Build history of the part. All positions in model axes, mm. A direction names the side the tool comes from. Give positions to 0.01 mm unless a question says otherwise; leave off trailing zeros. Order: outer loops, then holes, each group sorted by start corner. A loop starts at its lowest first (then second) coordinate and runs counter-clockwise, first axis right, second up. Notation, with made-up numbers: (-29, 29) - (-15, 29) arc R15 cw to (-15, 49) - close; hole circle Ø9 at (36, 83.25). An arc over 180 degrees is marked (long way). Use a Markdown table: item, result. Add a question column.
(1) Mould opens along X. For faces 1 (the face through (16, -100, 0)), 2 (the face through (-72.967, -66.909, -5.757)), 3 (the face through (47.53, 91.38, -6.26)) say: +X half, -X half, draft (parallel to the pull), parting line (faces both ways), or undercut.
(2) Which spindle directions (+Z, -Z, +X, -X, +Y, -Y) get a long thin tool onto all of the face, cutting with end or side? Do faces 4 (the face through (81, -52, 0)), 5 (the face through (97, -23, -11.356)). Say none if no direction does.
(3) Wall check: line 1 (Y direction, x = 0, z = -6.25); line 2 (Y direction, x = -72, z = -2.75); line 3 (X direction, y = -44.5, z = -1) (3 decimals). Give the ranges that are in metal, low to high.
(4) Flat gauge pins, fed straight in: pin 1 (8 mm diameter, centred on x = 60, z = -11, fed in from -Y); pin 2 (6 mm diameter, centred on x = 34, z = -2, fed in from +Y); pin 3 (8 mm diameter, centred on y = -42, z = -10, fed in from +X). Where does each tip first touch, or does it go through?
(5) Slice it at A-A (y = 0). Write the cut outline in (x, z).
(6) Slice it at C-C (z = -6.5). Write the cut outline in (x, y), then the cut area to 3 significant figures.
from build123d import *

# Parameters (mm, degrees)
FILLET2_R = 2
FILLET3_R = 2


with BuildPart() as part:
    # Sketch1 → Revolve1 (revolve)
    with BuildSketch(Plane(origin=(0, 0, 0), x_dir=(1, 0, 0), z_dir=(0, 1, 0)), mode=Mode.PRIVATE) as revolve1_sk:
        Polygon((-99, 0), (-99, 11.355578728), (-100, 11.355578728), (-100, 0), (-103, 0), (-103, 14.355578728), (-96, 14.355578728), (-96, 0), align=None)
    revolve(revolve1_sk.sketch.rotate(Axis((0, 0, 0), (0, 0, -1)), 180), axis=Axis((0, 0, 0), (0, 0, -1)))

    # Fillet2
    fillet2_edges = [part.edges().sort_by_distance(p)[0] for p in [
        (-103, 0, -14.355578728),
    ]]
    fillet(fillet2_edges, radius=FILLET2_R)

    # Fillet3
    fillet3_edges = [part.edges().sort_by_distance(p)[0] for p in [
        (-96, 0, -14.355578728),
    ]]
    fillet(fillet3_edges, radius=FILLET3_R)


solid = part.part
Solution:
| question | item | result |
|---|---|---|
| 1 | face 1 | draft |
| 1 | face 2 | undercut |
| 1 | face 3 | parting line |
| 2 | face 4 | +Z, +X, -X, +Y, -Y |
| 2 | face 5 | +Z |
| 3 | line 1 | -103 to -100, -99 to -96, 96 to 99, 100 to 103 |
| 3 | line 2 | -73.65 to -69.4, -67.95 to -63.5, 63.5 to 67.95, 69.4 to 73.65 |
| 3 | line 3 | -92.891 to -89.553, -88.435 to -85.063, 85.063 to 88.435, 89.553 to 92.891 |
| 4 | pin 1 | y = -86.45 |
| 4 | pin 2 | y = 98.22 |
| 4 | pin 3 | x = 95.73 |
| 5 | outline | (-103, -12.36) arc R2 ccw to (-101, -14.36) - (-98, -14.36) arc R2 ccw to (-96, -12.36) - (-96, 0) - (-99, 0) - (-99, -11.36) - (-100, -11.36) - (-100, 0) - (-103, 0) - close; (96, -12.36) arc R2 ccw to (98, -14.36) - (101, -14.36) arc R2 ccw to (103, -12.36) - (103, 0) - (100, 0) - (100, -11.36) - (99, -11.36) - (99, 0) - (96, 0) - close |
| 6 | outline | circle Ø206 at (0, 0); circle Ø198 at (0, 0); hole circle Ø200 at (0, 0); hole circle Ø192 at (0, 0) |
| 6 | area | 3,750 mm2 |
